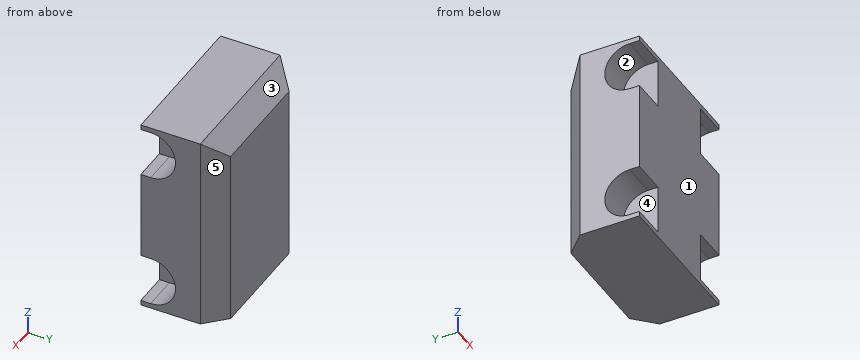
```python
from build123d import *

# Parameters (mm, degrees)
SKETCH1_W            = 150
SKETCH1_H            = 200
BOSS_EXTRUDE1_DEPTH  = 80
CUT_EXTRUDE3_DEPTH   = 35
MIRROR2_COPY_1_DEPTH = 35
CHAMFER1_SIZE        = 20


with BuildPart() as part:
    # Sketch1 → Boss-Extrude1 (new body)
    with BuildSketch(Plane(origin=(0, 0, 0), x_dir=(1, 0, 0), z_dir=(0, 1, 0))):
        Rectangle(SKETCH1_W, SKETCH1_H)
    extrude(amount=BOSS_EXTRUDE1_DEPTH)

    # Sketch4 → Cut-Extrude3 (cut)
    with BuildSketch(Plane.ZY.offset(75)):
        with BuildLine():
            Line((-92.912878475, 0), (-95, 0))
            Line((-95, 0), (-95, -15))
            Line((-95, -15), (-70, -15))
            ThreePointArc((-70, -15), (-83.693063938, -10.916500663), (-92.912878475, 0))
        make_face()
        with BuildLine():
            ThreePointArc((-92.912878475, 0), (-94.472657823, 4.892258908), (-95, 10))
            Line((-95, 10), (-95, 0))
            Line((-95, 0), (-92.912878475, 0))
        make_face()
        with BuildLine():
            Line((-45, 10), (-95, 10))
            ThreePointArc((-95, 10), (-94.472657823, 4.892258908), (-92.912878475, 0))
            Line((-92.912878475, 0), (-47.087121525, 0))
            ThreePointArc((-47.087121525, 0), (-45.527342177, 4.892258908), (-45, 10))
        make_face()
        with BuildLine():
            ThreePointArc((-45, 10), (-70, 35), (-95, 10))
            Line((-95, 10), (-45, 10))
        make_face()
        with BuildLine():
            Line((-45, 0), (-45, 10))
            ThreePointArc((-45, 10), (-45.527342177, 4.892258908), (-47.087121525, 0))
            Line((-47.087121525, 0), (-45, 0))
        make_face()
        with BuildLine():
            Line((-45, -15), (-45, 0))
            Line((-45, 0), (-47.087121525, 0))
            ThreePointArc((-47.087121525, 0), (-56.306936062, -10.916500663), (-70, -15))
            Line((-70, -15), (-45, -15))
        make_face()
        with BuildLine():
            Line((-47.087121525, 0), (-92.912878475, 0))
            ThreePointArc((-92.912878475, 0), (-83.693063938, -10.916500663), (-70, -15))
            ThreePointArc((-70, -15), (-56.306936062, -10.916500663), (-47.087121525, 0))
        make_face()
    cut_extrude3 = extrude(amount=-CUT_EXTRUDE3_DEPTH, mode=Mode.SUBTRACT)

    # Mirror1: Cut-Extrude3 across plane
    add(cut_extrude3.mirror(Plane.XY), mode=Mode.SUBTRACT)

    # Mirror2: Cut-Extrude3 across plane
    add(cut_extrude3.mirror(Plane.ZY), mode=Mode.SUBTRACT)

    # Mirror2 copy 1 sketch → Mirror2 copy 1 (cut)
    with BuildSketch(Plane(origin=(75, 0, 0), x_dir=(0, 0, -1), z_dir=(1, 0, 0))):
        with BuildLine():
            Line((-92.912878475, 0), (-95, 0))
            Line((-95, 0), (-95, -15))
            Line((-95, -15), (-70, -15))
            ThreePointArc((-70, -15), (-83.693063938, -10.916500663), (-92.912878475, 0))
        make_face()
        with BuildLine():
            ThreePointArc((-92.912878475, 0), (-94.472657823, 4.892258908), (-95, 10))
            Line((-95, 10), (-95, 0))
            Line((-95, 0), (-92.912878475, 0))
        make_face()
        with BuildLine():
            Line((-45, 10), (-95, 10))
            ThreePointArc((-95, 10), (-94.472657823, 4.892258908), (-92.912878475, 0))
            Line((-92.912878475, 0), (-47.087121525, 0))
            ThreePointArc((-47.087121525, 0), (-45.527342177, 4.892258908), (-45, 10))
        make_face()
        with BuildLine():
            ThreePointArc((-45, 10), (-70, 35), (-95, 10))
            Line((-95, 10), (-45, 10))
        make_face()
        with BuildLine():
            Line((-45, 0), (-45, 10))
            ThreePointArc((-45, 10), (-45.527342177, 4.892258908), (-47.087121525, 0))
            Line((-47.087121525, 0), (-45, 0))
        make_face()
        with BuildLine():
            Line((-45, -15), (-45, 0))
            Line((-45, 0), (-47.087121525, 0))
            ThreePointArc((-47.087121525, 0), (-56.306936062, -10.916500663), (-70, -15))
            Line((-70, -15), (-45, -15))
        make_face()
        with BuildLine():
            Line((-47.087121525, 0), (-92.912878475, 0))
            ThreePointArc((-92.912878475, 0), (-83.693063938, -10.916500663), (-70, -15))
            ThreePointArc((-70, -15), (-56.306936062, -10.916500663), (-47.087121525, 0))
        make_face()
    extrude(amount=-MIRROR2_COPY_1_DEPTH, mode=Mode.SUBTRACT)

    # Chamfer1
    chamfer1_edges = [part.edges().sort_by_distance(p)[0] for p in [
        (-75, 80, 0),
        (0, 80, 100),
        (75, 80, 0),
    ]]
    chamfer(chamfer1_edges, length=CHAMFER1_SIZE)


solid = part.part
```
Geometry: final body of the model. Coordinates: model frame, mm. Face numbers are marked on the shaded views. A direction names the side the tool comes from. Round coordinates to 2 decimals unless told otherwise and drop trailing zeros. Order: outer loops, then holes, each group sorted by start corner. A loop starts at its lowest first (then second) coordinate and runs counter-clockwise, first axis right, second up. Notation, with made-up numbers: (1, -6.75) -> (25, -6.75) arc R25 cw to (25, 27.25) -> close; hole circle Ø11 at (38, -14.5). An arc over 180 degrees is marked (long way). Use one line per item in the form item = value. Start each with the question number.
1. Cut plane B-B (x = 44). Return the cut outline in (y, z).
2. Pin query (flat end, axial travel): pin 1 Ø17.5 at (y, z) = (18, 72.5) entering from +X; pin 2 Ø10.5 at (y, z) = (16.5, 77) entering from -X. Return the tip coordinate at first contact, or that it passes through.
3. Line query: probe 1 along Z at (x, y) = (-48, 9.5); probe 2 along Z at (x, y) = (-63, 15); probe 3 along X at (y, z) = (75, 12). Output: solid intervals per line, ascending.
4. Reachability of the marked faces 1 and 2 from +Z, -Z, +X, -X, +Y, -Y: full face, straight path, thin tool, end or side. Return the list, or none.
5. Cut plane A-A (z = 70). Return the cut outline in (x, y), then the cut area to 3 significant figures.
6. Cut plane C-C (y = 25). Return the cut outline in (x, z).
7. Draft query along Z for the marked faces 3, 4 and 5. Return one class per face: pulls with the +Z half, pulls with the -Z half, needs draft (parallel to the pull), parting line crosses it, or undercut.
8. Cut plane D-D (z = -3). Return the cut outline in (x, y), then the cut area to 3 significant figures.
Solution:
q1.outline = (0, -100) -> (80, -100) -> (80, 80) -> (60, 100) -> (0, 100) -> (0, 95) -> (10, 95) arc R25 cw to (10, 45) -> (0, 45) -> (0, -45) -> (10, -45) arc R25 cw to (10, -95) -> (0, -95) -> close
q2.pin_1 = 40
q2.pin_2 = -40
q3.probe_1 = -100 to -95, -45 to 45, 95 to 100
q3.probe_2 = -100 to -94.49, -45.51 to 45.51, 94.49 to 100
q3.probe_3 = -60 to 60
q4.face_1 = +Z, -Z, +X, -X, -Y
q4.face_2 = -X, -Y
q5.outline = (-75, 35) -> (-40, 35) -> (-40, 0) -> (40, 0) -> (40, 35) -> (75, 35) -> (75, 60) -> (55, 80) -> (-55, 80) -> (-75, 60) -> close
q5.area = 9,150 mm^2
q6.outline = (-75, -100) -> (75, -100) -> (75, -90) -> (40, -90) -> (40, -50) -> (75, -50) -> (75, 50) -> (40, 50) -> (40, 90) -> (75, 90) -> (75, 100) -> (-75, 100) -> (-75, 90) -> (-40, 90) -> (-40, 50) -> (-75, 50) -> (-75, -50) -> (-40, -50) -> (-40, -90) -> (-75, -90) -> close
q7.face_3 = pulls with the +Z half
q7.face_4 = undercut
q7.face_5 = needs draft
q8.outline = (-75, 0) -> (75, 0) -> (75, 60) -> (55, 80) -> (-55, 80) -> (-75, 60) -> close
q8.area = 11,600 mm^2
